```python
from build123d import *

# Parameters (mm, degrees)
BOSS_EXTRUDE1_DEPTH = 55
SKETCH3_R           = 7.7
CUT_EXTRUDE1_DEPTH  = 2.8
SKETCH4_R           = 7.7
SKETCH4_R_2         = 5.5
BOSS_EXTRUDE2_DEPTH = 0.8
SKETCH5_W           = 15.4
SKETCH5_H           = 2
CUT_EXTRUDE2_DEPTH  = 8.5


with BuildPart() as part:
    # Sketch2 → Boss-Extrude1 (new body)
    with BuildSketch(Plane.XY):
        Polygon((2.6, -1.780794077), (19.6, -1.780794077), (19.6, 3.219205923), (22.2, 3.219205923), (22.2, 5.219205923), (0, 5.219205923), (0, 3.219205923), (2.6, 3.219205923), align=None)
    extrude(amount=-BOSS_EXTRUDE1_DEPTH)

    # Sketch3 → Cut-Extrude1 (cut)
    with BuildSketch(Plane.XZ.offset(1.780794077)):
        with Locations((11.1, -8.64)):
            Circle(SKETCH3_R)
        with Locations((11.1, -46.36)):
            Circle(SKETCH3_R)
    extrude(amount=-CUT_EXTRUDE1_DEPTH, mode=Mode.SUBTRACT)

    # Sketch4 → Boss-Extrude2 (add)
    with BuildSketch(Plane.XZ.offset(1.780794077)):
        with Locations((11.1, -8.64)):
            Circle(SKETCH4_R)
        with Locations((11.1, -8.64)):
            Circle(SKETCH4_R_2, mode=Mode.SUBTRACT)
        with Locations((11.1, -46.36)):
            Circle(SKETCH4_R)
        with Locations((11.1, -46.36)):
            Circle(SKETCH4_R_2, mode=Mode.SUBTRACT)
    extrude(amount=-BOSS_EXTRUDE2_DEPTH)

    # Sketch5 → Cut-Extrude2 (cut)
    with BuildSketch(Plane(origin=(19.6, 0, 0), x_dir=(0, 0, -1), z_dir=(1, 0, 0))):
        with Locations((8.64, 0.019205923)):
            Rectangle(SKETCH5_W, SKETCH5_H)
        with Locations((46.36, 0.719205923)):
            Rectangle(SKETCH5_W, SKETCH5_H)
    extrude(amount=-CUT_EXTRUDE2_DEPTH, mode=Mode.SUBTRACT)


solid = part.part
```
Input: part model. Units: mm. Frame: model coordinates. A direction names the side the tool comes from. Coordinates: 2 decimals unless noted, no trailing zeros. Loops run counter-clockwise (first coordinate to the right, second up) from the corner with the lowest first, then second, coordinate; pieces in that order, holes last. Notation, with made-up numbers: (29, 46.5) -> (57, 46.5) arc R21 cw to (57, 70.5) -> close; hole circle Ø4 at (57, 54.5). An arc over 180 degrees is marked (long way). Use a Markdown table: item, result.
1) Pull-direction query (Y, two-part tool) for faces 5 (the flat face through (21, 3.219, -27)), 6 (the flat face through (11, 5.219, -27)), 7 (the flat face through (11, 2, -55)), 8 (the flat face through (15, 0, -0.94)); classes: released by +Y, released by -Y, zero draft, split by the parting line, or undercut.
Results found:
| item | result |
|---|---|
| face 5 | released by -Y |
| face 6 | released by +Y |
| face 7 | zero draft |
| face 8 | undercut |
2) Cut plane D-D (x = 9.75). Return the cut outline in (y, z).
Results found:
| item | result |
|---|---|
| outline | (-1.78, -55) -> (5.22, -55) -> (5.22, 0) -> (-1.78, 0) -> (-1.78, -3.31) -> (-0.98, -3.31) -> (-0.98, -1.06) -> (1.02, -1.06) -> (1.02, -16.22) -> (-0.98, -16.22) -> (-0.98, -13.97) -> (-1.78, -13.97) -> (-1.78, -41.03) -> (-0.98, -41.03) -> (-0.98, -38.78) -> (1.02, -38.78) -> (1.02, -53.94) -> (-0.98, -53.94) -> (-0.98, -51.69) -> (-1.78, -51.69) -> close |
3) Cut plane C-C (z = -24.5). Return the cut outline in (x, y).
Results found:
| item | result |
|---|---|
| outline | (0, 3.22) -> (2.6, 3.22) -> (2.6, -1.78) -> (19.6, -1.78) -> (19.6, 3.22) -> (22.2, 3.22) -> (22.2, 5.22) -> (0, 5.22) -> close |
4) Cut plane A-A (z = -46.36). Return the cut outline in (x, y), then the cut area to 3 significant figures.
Results found:
| item | result |
|---|---|
| outline | (0, 3.22) -> (2.6, 3.22) -> (2.6, -1.78) -> (5.6, -1.78) -> (5.6, -0.98) -> (3.4, -0.98) -> (3.4, 1.02) -> (11.1, 1.02) -> (11.1, 1.72) -> (19.6, 1.72) -> (19.6, 3.22) -> (22.2, 3.22) -> (22.2, 5.22) -> (0, 5.22) -> close; (16.6, -1.78) -> (19.6, -1.78) -> (19.6, -0.28) -> (18.8, -0.28) -> (18.8, -0.98) -> (16.6, -0.98) -> close |
| area | 82.8 mm2 |
5) Material intervals for line 1 along Z through (x, y) = (15.25, -0.25); line 2 along Z through (x, y) = (11.1, -1.45); line 3 along Z through (x, y) = (15, 1.5), sorted ascending. Write a range as from..to.
Results found:
| item | result |
|---|---|
| line 1 | z = -55..-54.06, -38.66..-16.34, -0.94..0 |
| line 2 | z = -55..-51.86, -40.86..-14.14, -3.14..0 |
| line 3 | z = -55..-54.06, -38.66..0 |
6) Access query for faces 1 (the flat face through (11, 2, 0)), 2 (the flat face through (8, 1.019, -46)), 3 (the cylindrical face through (9.91, -1.39, -51.73)), 4 (the flat face through (2.6, 1, -27)). Directions: +Z, -Z, +X, -X, +Y, -Y. A direction counts if a zero-diameter tool reaches every point of the face in a straight line with its end or side. Return the directions, or none.
Results found:
| item | result |
|---|---|
| face 1 | +Z, +X, -X, +Y, -Y |
| face 2 | +X |
| face 3 | -Y |
| face 4 | +Z, -Z, -X, -Y |
7) Contact query for flat-ended pins moving along their axis: pin 1 (6.5 mm diameter, centred on x = 11.1, z = -8.64, fed in from -Y); pin 2 (4 mm diameter, centred on y = 0.5, z = -33.5, fed in from +X); pin 3 (3 mm diameter, centred on y = -0.5, z = -7, fed in from -X). Output: stop coordinate, or through.
Results found:
| item | result |
|---|---|
| pin 1 | stops at y = 1.02 |
| pin 2 | stops at x = 19.6 |
| pin 3 | stops at x = 2.6 |
8) Cut plane B-B (y = 0.25). Return the cut outline in (x, z), then the cut area to 3 significant figures.
Results found:
| item | result |
|---|---|
| outline | (2.6, -55) -> (19.6, -55) -> (19.6, -54.06) -> (11.1, -54.06) arc R7.7 cw to (11.1, -38.66) -> (19.6, -38.66) -> (19.6, -16.34) -> (11.1, -16.34) arc R7.7 cw to (11.1, -0.94) -> (19.6, -0.94) -> (19.6, 0) -> (2.6, 0) -> close |
| area | 487 mm2 |
